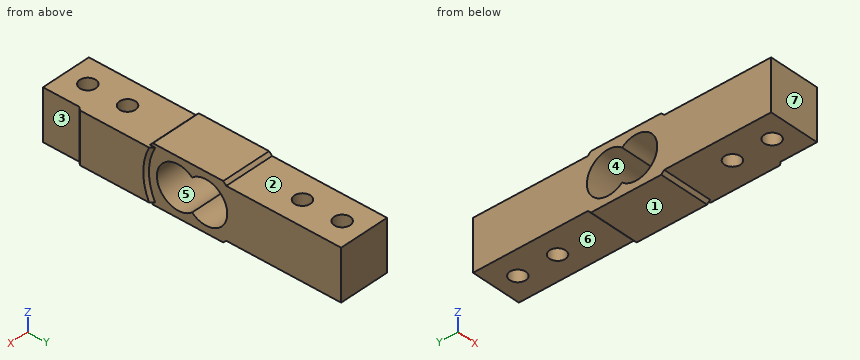
from build123d import *

# Parameters (mm, degrees)
SKETCH1_W               = 12.7
SKETCH1_H               = 12.7
BOSS_EXTRUDE1_DEPTH     = 37.5
CUT_EXTRUDE1_DEPTH      = 39.560277489
CUT_EXTRUDE1_DEPTH_BACK = 39.560277489
BOSS_EXTRUDE2_START     = -6.35
SKETCH3_W               = 0.75
SKETCH3_H               = 21.7
BOSS_EXTRUDE2_DEPTH     = 12.7
BOSS_EXTRUDE3_DEPTH     = 0.75
CHAMFER1_SIZE           = 2
CUT_EXTRUDE2_DEPTH      = 39.820999472
CUT_EXTRUDE2_DEPTH_BACK = 39.820999472
SKETCH5_R               = 2


with BuildPart() as part:
    # Sketch1 → Boss-Extrude1 (new, symmetric)
    with BuildSketch(Plane(origin=(0, 0, 0), x_dir=(1, 0, 0), z_dir=(0, 1, 0))):
        Rectangle(SKETCH1_W, SKETCH1_H)
    extrude(amount=BOSS_EXTRUDE1_DEPTH, both=True)

    # Sketch2 → Cut-Extrude1 (cut, two sides: drawn at the far end of the back side and taken through both)
    with BuildSketch(Plane(origin=(0, 0, 0), x_dir=(0, 0, -1), z_dir=(1, 0, 0)).offset(-CUT_EXTRUDE1_DEPTH_BACK)):
        with BuildLine():
            ThreePointArc((4.046294601, 0), (0, 8.85), (-4.046294601, 0))
            ThreePointArc((-4.046294601, 0), (0, -8.85), (4.046294601, 0))
        make_face()
    extrude(amount=CUT_EXTRUDE1_DEPTH + CUT_EXTRUDE1_DEPTH_BACK, mode=Mode.SUBTRACT)

    # Sketch3 → Boss-Extrude2 (add)
    with BuildSketch(Plane(origin=(0, 0, 0), x_dir=(0, 0, -1), z_dir=(1, 0, 0)).offset(BOSS_EXTRUDE2_START)):
        with Locations((6.725, -1)):
            Rectangle(SKETCH3_W, SKETCH3_H)
        with Locations((-6.725, -1)):
            Rectangle(SKETCH3_W, SKETCH3_H)
    extrude(amount=BOSS_EXTRUDE2_DEPTH)

    # Sketch4 → Boss-Extrude3 (add)
    with BuildSketch(Plane(origin=(6.35, 0, 0), x_dir=(0, 0, -1), z_dir=(1, 0, 0))):
        with BuildLine():
            Line((-6.35, -7.85), (-6.35, -29.55))
            Line((-6.35, -29.55), (6.35, -29.55))
            Line((6.35, -29.55), (6.35, -7.85))
            ThreePointArc((6.35, -7.85), (0, -9.6), (-6.35, -7.85))
        make_face()
    extrude(amount=BOSS_EXTRUDE3_DEPTH)

    # Chamfer1
    # the kernel refuses this chamfer: 2 mm, written as the material it takes off along each edge
    with BuildSketch(Plane(origin=(7.1, -29.55, 11.493365976), x_dir=(-0.9996219169112968, -0.027495876610585623, 0), z_dir=(0, 0, -1))) as chamfer1_piece_1_section:
        Polygon((CHAMFER1_SIZE * 0.999621916911, CHAMFER1_SIZE * 0.0274958766106), (-CHAMFER1_SIZE * 0.0274958766106, CHAMFER1_SIZE * 0.999621916911), (0, 0), align=None)
    chamfer1_piece_1 = extrude(amount=22.986731952, mode=Mode.PRIVATE)
    chamfer1_piece_1 = split(chamfer1_piece_1, bisect_by=Plane(origin=(6.35, -28.711332072, 0), z_dir=(1, 0, 0)), keep=Keep.TOP, mode=Mode.PRIVATE)
    add(chamfer1_piece_1, mode=Mode.SUBTRACT)
    with BuildSketch(Plane(origin=(7.1, 2.795714286, 0), x_dir=(0, -0.5793710900712427, -0.8150638870601863), z_dir=(0, 0.8150638870601863, -0.5793710900712427))) as chamfer1_piece_2_section:
        Polygon((12.395714286, CHAMFER1_SIZE), (12.395714286 + CHAMFER1_SIZE, 0), (12.395714286, 0), align=None)
    chamfer1_piece_2 = revolve(axis=Axis((7.1, 2.795714286, 0), (-1, 0, 0)), revolution_arc=109.187358772, mode=Mode.PRIVATE)
    chamfer1_piece_2 = split(chamfer1_piece_2, bisect_by=Plane(origin=(6.35, -11.230390822, 0), z_dir=(1, 0, 0)), keep=Keep.TOP, mode=Mode.PRIVATE)
    add(chamfer1_piece_2, mode=Mode.SUBTRACT)
    with BuildSketch(Plane(origin=(-11.493365976, -11.85, -7.1), x_dir=(0, 0.9996219169112968, -0.027495876610586487), z_dir=(1, 0, 0))) as chamfer1_piece_3_section:
        Polygon((CHAMFER1_SIZE * 0.999621916911, CHAMFER1_SIZE * 0.0274958766106), (-CHAMFER1_SIZE * 0.0274958766106, CHAMFER1_SIZE * 0.999621916911), (0, 0), align=None)
    chamfer1_piece_3 = extrude(amount=22.986731952, mode=Mode.PRIVATE)
    chamfer1_piece_3 = split(chamfer1_piece_3, bisect_by=Plane(origin=(0, -11.011332072, -6.35), z_dir=(0, 0, -1)), keep=Keep.TOP, mode=Mode.PRIVATE)
    add(chamfer1_piece_3, mode=Mode.SUBTRACT)
    with BuildSketch(Plane(origin=(-11.493365976, 9.85, -7.1), x_dir=(0, 0.027495876610586487, 0.9996219169112968), z_dir=(1, 0, 0))) as chamfer1_piece_4_section:
        Polygon((CHAMFER1_SIZE * 0.999621916911, CHAMFER1_SIZE * 0.0274958766106), (-CHAMFER1_SIZE * 0.0274958766106, CHAMFER1_SIZE * 0.999621916911), (0, 0), align=None)
    chamfer1_piece_4 = extrude(amount=22.986731952, mode=Mode.PRIVATE)
    chamfer1_piece_4 = split(chamfer1_piece_4, bisect_by=Plane(origin=(0, 9.011332072, -6.35), z_dir=(0, 0, -1)), keep=Keep.TOP, mode=Mode.PRIVATE)
    add(chamfer1_piece_4, mode=Mode.SUBTRACT)
    with BuildSketch(Plane(origin=(-11.493365976, 9.85, 7.1), x_dir=(0, -0.9996219169112968, 0.027495876610586497), z_dir=(1, 0, 0))) as chamfer1_piece_5_section:
        Polygon((CHAMFER1_SIZE * 0.999621916911, CHAMFER1_SIZE * 0.0274958766106), (-CHAMFER1_SIZE * 0.0274958766106, CHAMFER1_SIZE * 0.999621916911), (0, 0), align=None)
    chamfer1_piece_5 = extrude(amount=22.986731952, mode=Mode.PRIVATE)
    chamfer1_piece_5 = split(chamfer1_piece_5, bisect_by=Plane(origin=(0, 9.011332072, 6.35), z_dir=(0, 0, 1)), keep=Keep.TOP, mode=Mode.PRIVATE)
    add(chamfer1_piece_5, mode=Mode.SUBTRACT)
    with BuildSketch(Plane(origin=(-11.493365976, -11.85, 7.1), x_dir=(0, -0.027495876610586487, -0.9996219169112968), z_dir=(1, 0, 0))) as chamfer1_piece_6_section:
        Polygon((CHAMFER1_SIZE * 0.999621916911, CHAMFER1_SIZE * 0.0274958766106), (-CHAMFER1_SIZE * 0.0274958766106, CHAMFER1_SIZE * 0.999621916911), (0, 0), align=None)
    chamfer1_piece_6 = extrude(amount=22.986731952, mode=Mode.PRIVATE)
    chamfer1_piece_6 = split(chamfer1_piece_6, bisect_by=Plane(origin=(0, -11.011332072, 6.35), z_dir=(0, 0, 1)), keep=Keep.TOP, mode=Mode.PRIVATE)
    add(chamfer1_piece_6, mode=Mode.SUBTRACT)

    # Sketch5 → Cut-Extrude2 (cut, two sides: drawn at the far end of the back side and taken through both)
    with BuildSketch(Plane.XY.offset(-CUT_EXTRUDE2_DEPTH_BACK)):
        with Locations((0, 32)):
            Circle(SKETCH5_R)
        with Locations((0, 22)):
            Circle(SKETCH5_R)
        with Locations((0, -32)):
            Circle(SKETCH5_R)
        with Locations((0, -22)):
            Circle(SKETCH5_R)
    extrude(amount=CUT_EXTRUDE2_DEPTH + CUT_EXTRUDE2_DEPTH_BACK, mode=Mode.SUBTRACT)


solid = part.part
The listing builds one solid part. Answer for the finished solid, in the listing's coordinates (mm). Face numbers are marked on the shaded views. A direction names the side the tool comes from. Coordinates: 2 decimals unless noted, no trailing zeros. Write each loop counter-clockwise with the first axis right and the second up, starting at its lowest first coordinate (ties: lowest second). Pieces come first, ordered by that corner, then holes. Notation, with made-up numbers: (88.25, -15.75) - (135.25, -15.75) arc R23 ccw to (135.25, 1.25) - close; hole circle Ø2 at (66.5, -36.5). An arc over 180 degrees is marked (long way). Return JSON: item names as keys, results as strings.
1. Which of the six approach directions +Z, -Z, +X, -X, +Y, -Y give full straight-line access (tool end or side, diameter ignored) to the marked faces 1, 2 and 3?
Final values:
{"face 1": "-Z, +X, -X, +Y, -Y", "face 2": "+Z, +X, -X, +Y", "face 3": "+Z, -Z, +X, -Y"}
2. Each of these flat-tipped pins is pushed along its axis until it touches: pin 1 Ø6.5 at (x, y) = (-2, 19.5) entering from +Z; pin 2 Ø4.5 at (y, z) = (11.5, 2) entering from +X; pin 3 Ø8.5 at (y, z) = (3.5, 0) entering from -X; pin 4 Ø5 at (x, y) = (0, -22) entering from -Z. Where does it stop, or does it pass through?
Final values:
{"pin 1": "z = 6.35", "pin 2": "x = 6.35", "pin 3": "through", "pin 4": "z = -6.35"}
3. Consider line 1 along Y through (x, z) = (0, 0); line 2 along Y through (x, z) = (0, 4); line 3 along Y through (x, z) = (-1.5, -6). Determine where each line is inside the solid, lowest interval first.
Final values:
{"line 1": "-37.5 to -34, -30 to -24, -20 to -8.85, 8.85 to 20, 24 to 30, 34 to 37.5", "line 2": "-37.5 to -34, -30 to -24, -20 to -7.05, 7.05 to 20, 24 to 30, 34 to 37.5", "line 3": "-37.5 to -33.32, -30.68 to -23.32, -20.68 to 20.68, 23.32 to 30.68, 33.32 to 37.5"}
4. For a pull along Y with two mould halves and no side action, classify the marked faces 4, 5, 6 and 7 as +Y half, -Y half, draft (parallel to the pull), parting line (faces both ways), or undercut.
Final values:
{"face 4": "undercut", "face 5": "undercut", "face 6": "draft", "face 7": "-Y half"}
5. The part is cut by section A-A on y = -3.5. Determine the outline of the cut face in (x, z).
Final values:
{"outline": "(-6.35, -7.1) - (6.35, -7.1) - (6.35, -5.35) - (-6.35, -5.35) - close; (-6.35, 5.35) - (6.35, 5.35) - (6.35, 7.1) - (-6.35, 7.1) - close"}
6. The part is cut by section D-D on y = 22. Determine the outline of the cut face in (x, z), then the cut area to 3 significant figures.
Final values:
{"outline": "(-6.35, -6.35) - (-2, -6.35) - (-2, 6.35) - (-6.35, 6.35) - close; (2, -6.35) - (6.35, -6.35) - (6.35, 6.35) - (2, 6.35) - close", "area": "110 mm^2"}
7. The part is cut by section B-B on z = 0. Determine the outline of the cut face in (x, y), then the cut area to 3 significant figures.
Final values:
{"outline": "(-6.35, -37.5) - (6.35, -37.5) - (6.35, -28.3) - (7.1, -27.55) - (7.1, -11.6) - (6.35, -10.85) - (6.35, -8.85) - (-6.35, -8.85) - close; (-6.35, 8.85) - (6.35, 8.85) - (6.35, 37.5) - (-6.35, 37.5) - close; hole circle Ø4 at (0, -32); hole circle Ø4 at (0, -22); hole circle Ø4 at (0, 22); hole circle Ø4 at (0, 32)", "area": "690 mm^2"}
8. The part is cut by section C-C on x = -0.5. Count the separate pieces of the cut face and the enclosed holes in it, then the cut area to 3 significant figures.
Final values:
{"separate pieces": "5", "enclosed holes": "1", "area": "624 mm^2"}
